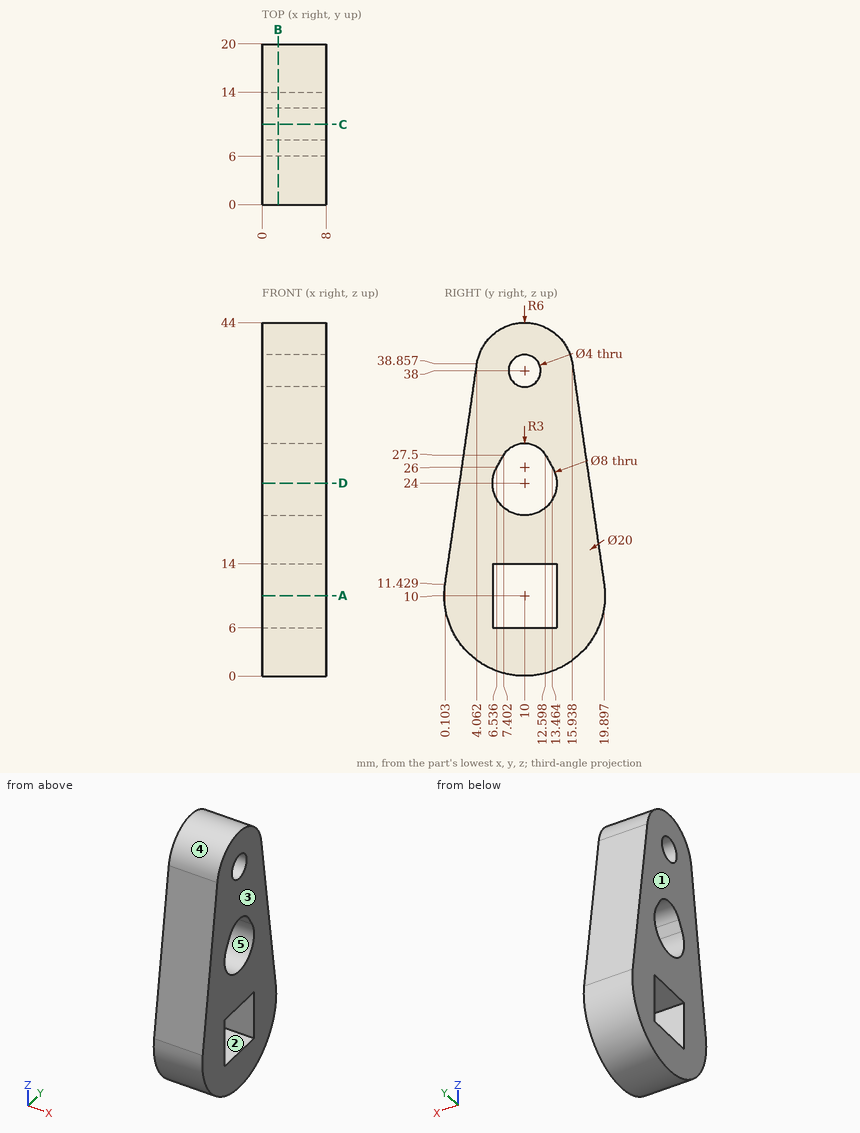
Input: dimensioned drawing with shaded views. Units: mm. Origin: part minimum x, y, z. A direction names the side the tool comes from. Coordinates: 2 decimals unless noted, no trailing zeros. Write each loop counter-clockwise with the first axis right and the second up, starting at its lowest first coordinate (ties: lowest second). Pieces come first, ordered by that corner, then holes. Notation, with made-up numbers: M -19.5,-12 L -12.5,-12 A21 ccw -12.5,17 Z; hole C 52,-35 d5. An arc over 180 degrees is marked long. Answer as CSV lines item,"result". Start each with the question number.
Q1. Mould query, pull axis Y, two halves, no side actions, for the marked faces 3, 4 and 5. Classes: released by +Y, released by -Y, zero draft, split by the parting line, or undercut.
Q2. Reachability of the marked faces 1 and 2 from +Z, -Z, +X, -X, +Y, -Y: full face, straight path, thin tool, end or side. Return the list, or none.
Q3. Cut plane C-C on y = 10. Return the cut outline in (x, z), then the cut area to 3 significant figures.
Q4. Pin query (flat end, axial travel): P1, Ø1.5, axis at x = 1.5, y = 5, coming from the +Z side (1 decimal); P2, Ø1, axis at x = 3, z = 16.5, coming from the +Y side; P3, Ø4, axis at x = 5, z = 30.5, coming from the -Y side. Return the tip coordinate at first contact, or that it passes through.
Q5. Cut plane B-B on x = 2. Return the cut outline in (y, z) (1 decimal).
Q6. Cut plane D-D on z = 24. Return the cut outline in (x, y).
Q7. Cut plane A-A on z = 10. Return the cut outline in (x, y).
Q8. Line query: line 1 (Z direction, x = 4.25, y = 10); line 2 (Z direction, x = 4.75, y = 6.5) (1 decimal); line 3 (Y direction, x = 4.5, z = 38). Output: solid intervals per line, ascending. Write a range as from..to.
Findings below:
1,face 3,"zero draft"
1,face 4,"split by the parting line"
1,face 5,"undercut"
2,face 1,"+Z, -Z, -X, +Y, -Y"
2,face 2,"+X, -X"
3,outline,"M 0,0 L 8,0 L 8,6 L 0,6 Z; M 0,14 L 8,14 L 8,20 L 0,20 Z; M 0,29 L 8,29 L 8,36 L 0,36 Z; M 0,40 L 8,40 L 8,44 L 0,44 Z"
3,area,"184 mm2"
4,P1,"stops at z = 42.2"
4,P2,"stops at y = 19.24"
4,P3,"stops at y = 2.57"
5,outline,"M 0.1,11.4 A10 ccw long 19.9,11.4 L 15.9,38.9 A6 ccw 4.1,38.9 Z; hole M 6,6 L 14,6 L 14,14 L 6,14 Z; hole M 6.5,26 A4 ccw long 13.5,26 L 12.6,27.5 A3 ccw 7.4,27.5 Z; hole C 10,38 d4"
6,outline,"M 0,1.92 L 8,1.92 L 8,6 L 0,6 Z; M 0,14 L 8,14 L 8,18.08 L 0,18.08 Z"
7,outline,"M 0,0 L 8,0 L 8,6 L 0,6 Z; M 0,14 L 8,14 L 8,20 L 0,20 Z"
8,line 1,"z = 0..6, 14..20, 29..36, 40..44"
8,line 2,"z = 0.6..6, 14..22.1, 25.9..42.9"
8,line 3,"y = 3.94..8, 12..16.06"
